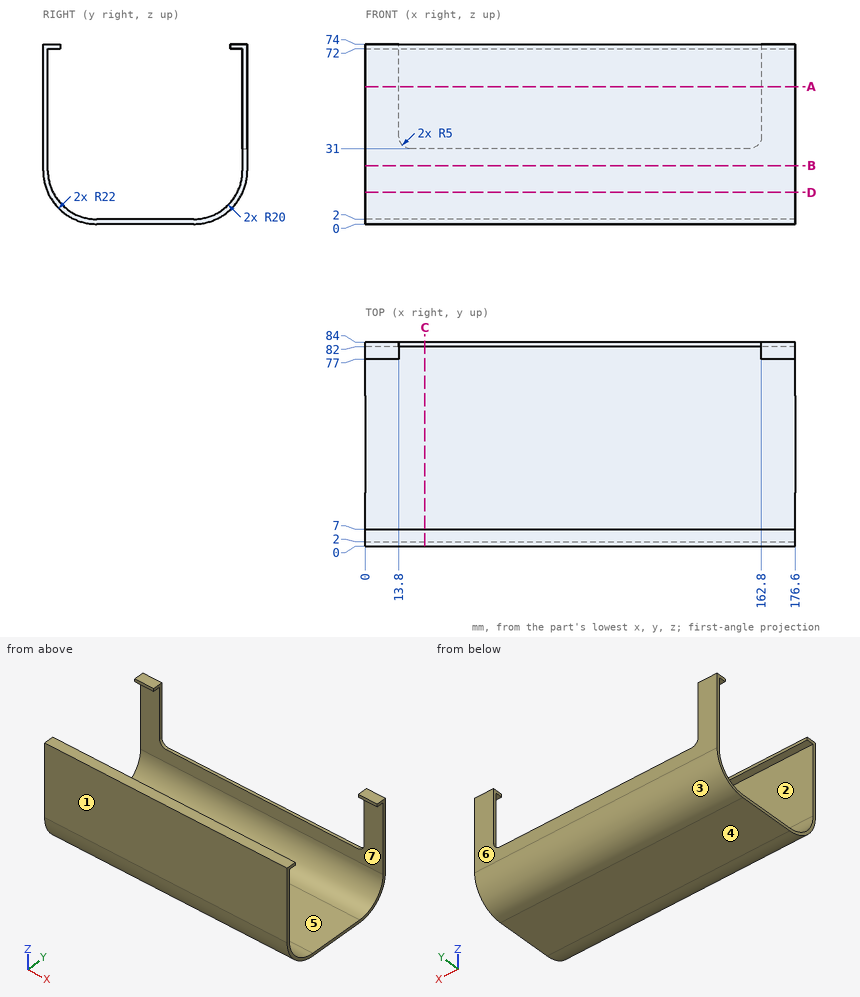
Here's the drawing with two shaded views (mm, measured from the low corner). I have some questions. A direction names the side the tool comes from. Round coordinates to 2 decimals unless told otherwise and drop trailing zeros. Write each loop counter-clockwise with the first axis right and the second up, starting at its lowest first coordinate (ties: lowest second). Pieces come first, ordered by that corner, then holes. Notation, with made-up numbers: M 88,-32 L 144,-32 A30 cw 144,4 Z; hole C -13.75,-17 d1. An arc over 180 degrees is marked long. Write each question's results on one line, items separated by ' | '. Start each with the question number.
1. I need wall thicknesses on L1, parallel to Y at x = 114.5, z = 29; L2, parallel to Y at x = 138.5, z = 60. Which ranges of each line are inside material? Lowest first, please. Write a range as from..to.
2. Imagine slicing it at C-C on x = 24.5. List the corners of the cut face in (y, z) for me.
3. Thinking about a two-plate mould opening in Y: for the marked faces 1, 2, 3 and 4, which applies, +Y half, -Y half, draft (parallel to the pull), parting line (faces both ways), or undercut?
4. Imagine slicing it at D-D on z = 13. List the corners of the cut face in (x, y) for me, and give its area (3 significant figures).
5. Imagine slicing it at A-A on z = 56.5. List the corners of the cut face in (x, y) for me.
6. On a 3-axis mill with a long thin cutter (end or side, diameter ignored), from which of +Z, -Z, +X, -X, +Y, -Y can I reach the whole of each face in a straight line? I mean the marked faces 5, 6 and 7. Say none if no direction works.
7. Imagine slicing it at B-B on z = 24. List the corners of the cut face in (x, y) for me.
8. I'm going to push flat-ended pins straight in: pin 1 Ø12 at (x, y) = (61, 11) entering from -Z; pin 2 Ø5.5 at (x, y) = (9, 79) entering from -Z; pin 3 Ø3 at (x, y) = (86, 71.5) entering from +Z. Where does each tip first touch, or does it pass through?
Result sheet:
1) L1: y = 0..2, 82..84 | L2: y = 0..2
2) outline: M 0,22 A22 ccw 22,0 L 62,0 A22 ccw 84,22 L 84,31 L 82,31 L 82,22 A20 cw 62,2 L 22,2 A20 cw 2,22 L 2,72 L 7,72 L 7,74 L 0,74 Z
3) face 1: -Y half | face 2: undercut | face 3: +Y half | face 4: draft
4) outline: M 0,1.93 L 176.6,1.93 L 176.6,4.14 L 0,4.14 Z; M 0,79.86 L 176.6,79.86 L 176.6,82.07 L 0,82.07 Z | area: 782 mm^2
5) outline: M 0,0 L 176.6,0 L 176.6,2 L 0,2 Z; M 0,82 L 13.8,82 L 13.8,84 L 0,84 Z; M 162.8,82 L 176.6,82 L 176.6,84 L 162.8,84 Z
6) face 5: +Z, +X, -X | face 6: +Z, -Z, +X, -X, +Y | face 7: +X, -X
7) outline: M 0,0 L 176.6,0 L 176.6,2 L 0,2 Z; M 0,82 L 176.6,82 L 176.6,84 L 0,84 Z
8) pin 1: stops at z = 0.58 | pin 2: stops at z = 5.24 | pin 3: stops at z = 5.3
